Read the model definition and answer for the solid it produces. Units are mm, in the model's axes. A direction names the side the tool comes from. Coordinates: 2 decimals unless noted, no trailing zeros. Loops run counter-clockwise (first coordinate to the right, second up) from the corner with the lowest first, then second, coordinate; pieces in that order, holes last. Notation, with made-up numbers: (4, -3) - (35, -3) arc R17 cw to (35, 12) - close; hole circle Ø10 at (9, -27.75). An arc over 180 degrees is marked (long way). Use one line per item in the form item = value. Start each with the question number.
1) Consider line 1 (Z direction, x = -2, y = -3); line 2 (Y direction, x = 0.5, z = 6); line 3 (X direction, y = 2.25, z = 38.5). Determine where each line is inside the solid, lowest interval first.
2) Each of these flat-tipped pins is pushed along its axis until it touches: P1, Ø4, axis at x = 0, z = 27.5, coming from the +Y side; P2, Ø1.5, axis at y = -0.5, z = 11, coming from the +X side; P3, Ø1.5, axis at x = 3.5, z = 31.5, coming from the -Y side. Where does it stop, or does it pass through?
3) A cutting plane is placed at C-C (z = 5.5). Give the vertices of the cut face in (x, y).
4) Which of the six approach directions +Z, -Z, +X, -X, +Y, -Y give full straight-line access (tool end or side, diameter ignored) to faces 1 (the face through (-3, 0, 20)), 2 (the face through (3.164, -3.2, 41.479))?
5) A cutting plane is placed at A-A (x = 0). Give the vertices of the cut face in (y, z), and give its area (3 significant figures).
from build123d import *

# Parameters (mm, degrees)
SKETCH1_R           = 3
BOSS_EXTRUDE1_DEPTH = 40
BOSS_EXTRUDE2_DEPTH = 3


with BuildPart() as part:
    # Sketch1 → Boss-Extrude1 (new body)
    with BuildSketch(Plane.XY):
        Circle(SKETCH1_R)
    extrude(amount=BOSS_EXTRUDE1_DEPTH)

    # Sketch2 → Boss-Extrude2 (add)
    with BuildSketch(Plane.XY.offset(40)):
        Polygon((-1.863961031, -4.5), (1.863961031, -4.5), (4.5, -1.863961031), (4.5, 1.863961031), (1.863961031, 4.5), (-1.863961031, 4.5), (-4.5, 1.863961031), (-4.5, -1.863961031), align=None)
    extrude(amount=BOSS_EXTRUDE2_DEPTH)


solid = part.part
Found:
q1.line_1 = 40 to 43
q1.line_2 = -2.96 to 2.96
q1.line_3 = -1.98 to 1.98
q2.P1 = 3
q2.P2 = 3
q2.P3 = -1.2
q3.outline = circle Ø6 at (0, 0)
q4.face_1 = -Z
q4.face_2 = +Z, -Z, +X, -Y
q5.outline = (-4.5, 40) - (-3, 40) - (-3, 0) - (3, 0) - (3, 40) - (4.5, 40) - (4.5, 43) - (-4.5, 43) - close
q5.area = 267 mm^2
